Geometry: final body of the model. Coordinates: model frame, mm. A direction names the side the tool comes from. Give positions to 0.01 mm unless a question says otherwise; leave off trailing zeros. Loops run counter-clockwise (first coordinate to the right, second up) from the corner with the lowest first, then second, coordinate; pieces in that order, holes last.
1. Material intervals for line 1 along Z through (x, y) = (8.5, 5); line 2 along Z through (x, y) = (1.75, -3); line 3 along X through (y, z) = (3, 20), sorted ascending.
2. Section D-D, the plane x = -3.5. Output: boundary loops of the cut face in (y, z), then the cut area to 3 significant figures.
3. Section A-A, the plane x = 0. Output: boundary loops of the cut face in (y, z), then the cut area to 3 significant figures.
4. First-contact query: P1, Ø12, axis at x = -8.5, z = 44.5, coming from the +Y side; P2, Ø6, axis at x = -5.5, z = 41, coming from the -Y side; P3, Ø1, axis at x = 6.5, z = 21, coming from the -Y side. Flat tips, straight axial feed; report the tip coordinate or a pass-through.
5. Section C-C, the plane z = 18.5. Output: boundary loops of the cut face in (x, y), then the cut area to 3 significant figures.
6. Access query for faces 1 (the face through (-0.1, -3.3, 39.2)), 2 (the face through (0, 0, 10.7)). Directions: +Z, -Z, +X, -X, +Y, -Y. A direction counts if a zero-diameter tool reaches every point of the face in a straight line with its end or side. Return the directions, or none.
from build123d import *

# Parameters (mm, degrees)
CYLINDER053_R     = 5
CYLINDER053_DEPTH = 9
CYLINDER054_R     = 3
CYLINDER054_DEPTH = 11.4
CYLINDER052_R     = 10.75
CYLINDER052_DEPTH = 19.5


with BuildPart() as pot_thread:
    # Cylinder053 → Cylinder053 (new body)
    with BuildSketch(Plane.XY.offset(19.5)):
        Circle(CYLINDER053_R)
    extrude(amount=CYLINDER053_DEPTH)


with BuildPart() as pot_axis:
    # Cylinder054 → Cylinder054 (new body)
    with BuildSketch(Plane.XY.offset(28.5)):
        Circle(CYLINDER054_R)
    extrude(amount=CYLINDER054_DEPTH)


with BuildPart() as obj1:
    # Cylinder052 → Cylinder052 (new body)
    with BuildSketch(Plane.XY):
        Circle(CYLINDER052_R)
    extrude(amount=CYLINDER052_DEPTH)

    # Fusion024: union pot-thread, pot-axis
    add(pot_thread.part)
    add(pot_axis.part)


with BuildPart() as obj1_1:
    # Fusion024 placement: moved
    add(obj1.part.moved(Location((0, 0, 10.7))))


solid = obj1_1.part
Answers below:
1. line 1: z = 10.7 to 30.2
1. line 2: z = 10.7 to 39.2
1. line 3: x = -10.32 to 10.32
2. outline: (-10.16, 10.7) - (10.16, 10.7) - (10.16, 30.2) - (3.57, 30.2) - (3.57, 39.2) - (-3.57, 39.2) - (-3.57, 30.2) - (-10.16, 30.2) - close
2. area: 461 mm2
3. outline: (-10.75, 10.7) - (10.75, 10.7) - (10.75, 30.2) - (5, 30.2) - (5, 39.2) - (3, 39.2) - (3, 50.6) - (-3, 50.6) - (-3, 39.2) - (-5, 39.2) - (-5, 30.2) - (-10.75, 30.2) - close
3. area: 578 mm2
4. P1: stops at y = 1.66
4. P2: stops at y = -3.92
4. P3: stops at y = -8.92
5. outline: circle Ø21.5 at (0, 0)
5. area: 363 mm2
6. face 1: +Z
6. face 2: -Z, +X, -X, +Y, -Y
